from build123d import *

# Parameters (mm, degrees)
SKETCH1_W           = 3.81
SKETCH1_H           = 12.7
SKETCH2_R           = 1.778
CUT_EXTRUDE1_DEPTH  = 4.81
SKETCH3_OUTSIDE_W   = 239.386
SKETCH3_OUTSIDE_H   = 239.386
CUT_EXTRUDE15_DEPTH = 4.81
CUT_EXTRUDE15_TAPER = 1
SKETCH8_W           = 7.62
SKETCH8_H           = 3.81
BOSS_EXTRUDE1_DEPTH = 10.922
CUT_EXTRUDE16_DEPTH = 6.096


with BuildPart() as part:
    # Sketch1 → Revolve1 (revolve)
    with BuildSketch(Plane(origin=(0, 0, 0), x_dir=(0, 0, -1), z_dir=(1, 0, 0)), mode=Mode.PRIVATE) as revolve1_sk:
        with Locations((-1.905, 86.106)):
            Rectangle(SKETCH1_W, SKETCH1_H)
    revolve(revolve1_sk.sketch.rotate(Axis((0, 0, 0), (0, 0, -1)), 90), axis=Axis((0, 0, 0), (0, 0, -1)))  # turned: the seam where the file's is

    # Sketch2 → Cut-Extrude1 (cut, through all)
    with BuildSketch(Plane.XY.offset(3.81)):
        with Locations((0, 87.376)):
            Circle(SKETCH2_R)
        with Locations((68.313308, 54.478045)):
            Circle(SKETCH2_R)
        with Locations((85.185301, -19.442989)):
            Circle(SKETCH2_R)
        with Locations((37.911026, -78.723056)):
            Circle(SKETCH2_R)
        with Locations((-37.911026, -78.723056)):
            Circle(SKETCH2_R)
        with Locations((-85.185301, -19.442989)):
            Circle(SKETCH2_R)
        with Locations((-68.313308, 54.478045)):
            Circle(SKETCH2_R)
    extrude(amount=-CUT_EXTRUDE1_DEPTH, mode=Mode.SUBTRACT)

    # Sketch3 outside → Cut-Extrude15 (cut, through all)
    with BuildSketch(Plane.XY.offset(3.81)):
        Rectangle(SKETCH3_OUTSIDE_W, SKETCH3_OUTSIDE_H)
        with BuildLine():
            ThreePointArc((-46.620921, -64.710967), (-55.484924, -66.151258), (-54.044634, -75.015262))
            ThreePointArc((-54.044634, -75.015262), (0, -92.456), (54.044634, -75.015262))
            ThreePointArc((54.044634, -75.015262), (55.484924, -66.151258), (46.620921, -64.710967))
            ThreePointArc((46.620921, -64.710967), (0, -79.756), (-46.620921, -64.710967))
        make_face(mode=Mode.SUBTRACT)
        with BuildLine():
            ThreePointArc((-52.63259, -71.960032), (-38.682471, -80.324978), (-23.444735, -86.016162))
            ThreePointArc((-23.444735, -86.016162), (-21.261754, -84.768299), (-22.509617, -82.585318))
            ThreePointArc((-22.509617, -82.585318), (-37.13958, -77.121133), (-50.533285, -69.089831))
            ThreePointArc((-50.533285, -69.089831), (-53.018038, -69.475278), (-52.63259, -71.960032))
        make_face()
        with BuildLine():
            ThreePointArc((23.563518, -86.016162), (38.801254, -80.324978), (52.751374, -71.960032))
            ThreePointArc((52.751374, -71.960032), (53.136821, -69.475278), (50.652068, -69.089831))
            ThreePointArc((50.652068, -69.089831), (37.258363, -77.121133), (22.6284, -82.585318))
            ThreePointArc((22.6284, -82.585318), (21.380537, -84.768299), (23.563518, -86.016162))
        make_face()
    extrude(amount=-CUT_EXTRUDE15_DEPTH, taper=CUT_EXTRUDE15_TAPER, mode=Mode.SUBTRACT)

    # Sketch8 → Boss-Extrude1 (add)
    with BuildSketch(Plane.XZ.offset(79.756)):
        with Locations((0, 1.905)):
            Rectangle(SKETCH8_W, SKETCH8_H)
    extrude(amount=-BOSS_EXTRUDE1_DEPTH)

    # Sketch9 → Cut-Extrude16 (cut)
    with BuildSketch(Plane(origin=(0, -68.834, 0), x_dir=(1, 0, 0), z_dir=(0, 1, 0))):
        Polygon((1.27, 0), (-1.27, 0), (-2.032, -0.635), (-2.032, -1.651), (2.032, -1.651), (2.032, -0.635), align=None)
    extrude(amount=-CUT_EXTRUDE16_DEPTH, mode=Mode.SUBTRACT)


solid = part.part
Input: part model. Units: mm. Frame: model coordinates. A direction names the side the tool comes from. Give positions to 0.01 mm unless a question says otherwise; leave off trailing zeros. Write each loop counter-clockwise with the first axis right and the second up, starting at its lowest first coordinate (ties: lowest second). Pieces come first, ordered by that corner, then holes. Notation, with made-up numbers: M 51,88 L 77,88 A26 cw 77,110 Z; hole C 70.5,-31.75 d2. An arc over 180 degrees is marked long. Write item = value, one per line. Start each with the question number.
1) Draft query along X for faces 1 (the cylindrical face through (0.821, -92.452, 1.878)), 2 (the cylindrical face through (-26.41, -75.257, 1.878)), 3 (the flat face through (-1, -81, 0)). Return one class per face: +X half, -X half, draft (parallel to the pull), parting line (faces both ways), or undercut.
2) Reachability of faces 4 (the flat face through (3.81, -74, 2)), 5 (the flat face through (1, -81, 3.81)), 6 (the flat face through (0, -72, 1.651)) from +Z, -Z, +X, -X, +Y, -Y: full face, straight path, thin tool, end or side. Return the list, or none.
3) Cut plane D-D on y = -89.25. Return the cut outline in (x, z).
4) Cut plane C-C on x = -5. Return the cut outline in (y, z), then the cut area to 3 significant figures.
5) Material intervals for line 1 along Y through (x, z) = (43, 0.9); line 2 along Y through (x, z) = (-31, 2.75); line 3 along X through (y, z) = (-71.5, 2.95), sorted ascending. Write a range as [from, to].
6) First-contact query: pin 1 Ø1.1 at (y, z) = (-74.5, 1) entering from -X; pin 2 Ø0.5 at (x, z) = (-0.5, 0.5) entering from +Y; pin 3 Ø0.8 at (y, z) = (-70.5, 1.5) entering from -X. Flat tips, straight axial feed; report the tip coordinate or a pass-through.
7) Cut plane A-A on z = 3.1. Count the separate pieces of the cut face and the enclosed holes in it, then the cut area to 3 significant figures.
Solved:
q1.face_1 = parting line
q1.face_2 = undercut
q1.face_3 = draft
q2.face_4 = +Z, -Z, +Y
q2.face_5 = +Z, +X, -X, +Y, -Y
q2.face_6 = +Y
q3.outline = M -24.14,0 L 24.14,0 L 24.14,3.81 L -24.14,3.81 Z
q4.outline = M -92.32,0 L -79.6,0 L -79.6,3.81 L -92.32,3.81 Z
q4.area = 48.5 mm2
q5.line_1 = [-81.85, -78.11], [-74.14, -67.17]
q5.line_2 = [-87.1, -83.57], [-79.81, -73.48]
q5.line_3 = [-56.48, -53.05], [-47.09, -35.34], [-3.81, 3.81], [35.34, 47.21], [53.17, 56.48]
q6.pin_1 = -55.26
q6.pin_2 = -74.93
q6.pin_3 = -56.72
q7.separate_pieces = 1
q7.enclosed_holes = 2
q7.area = 1,330 mm2
